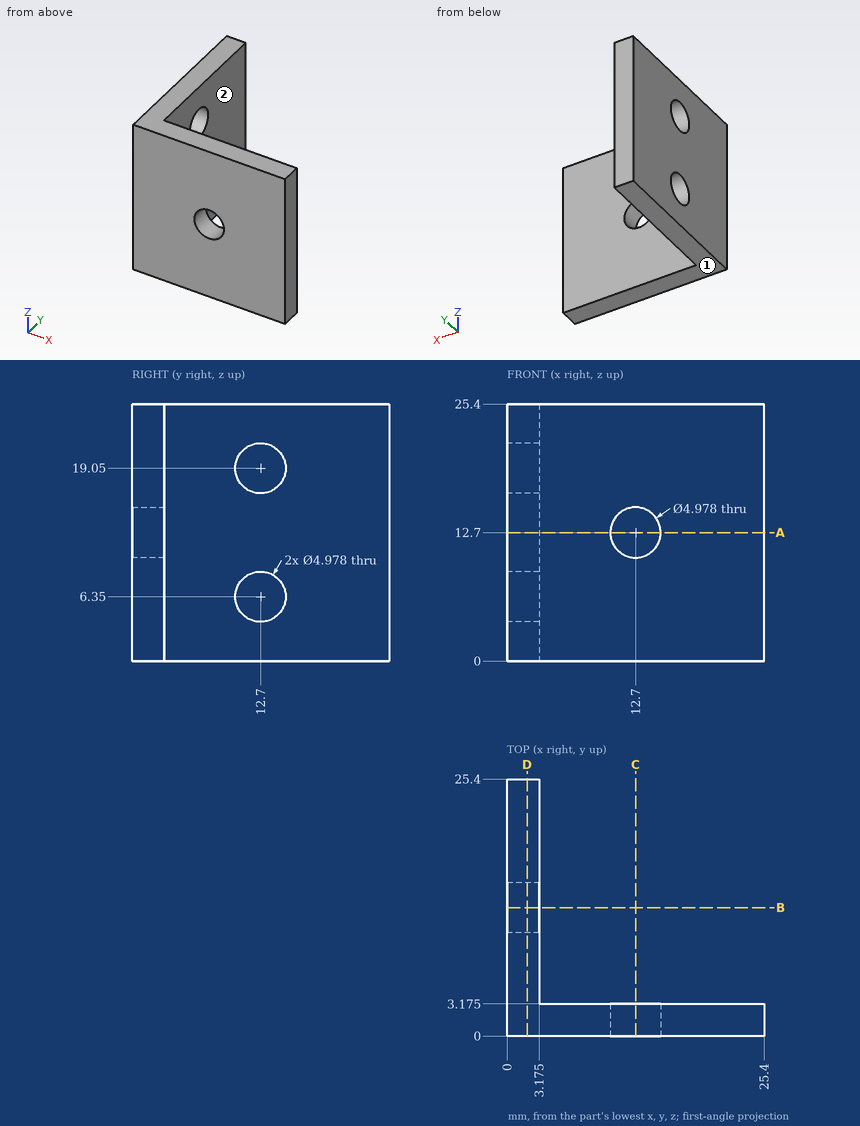
Study the drawing (mm; zero at the part's minimum x, y, z) and answer. A direction names the side the tool comes from. Coordinates: 2 decimals unless noted, no trailing zeros. Loops run counter-clockwise (first coordinate to the right, second up) from the corner with the lowest first, then second, coordinate; pieces in that order, holes last. Notation, with made-up numbers: (-35.5, -5) -> (-6.5, -5) arc R24 cw to (-6.5, 6) -> close; hole circle Ø4 at (15, 49). An arc over 180 degrees is marked (long way). Answer as CSV lines item,"result".
1) Straight lines are drawn through the part: probe 1 along Z at (x, y) = (2.55, 12.7); probe 2 along X at (y, z) = (0.9, 12.7). For each, find the intervals that lie inside material, in ascending order.
A:
probe 1,"z = 0 to 3.86, 8.84 to 16.56, 21.54 to 25.4"
probe 2,"x = 0 to 10.21, 15.19 to 25.4"
2) The part is cut by section D-D (x = 2). Give the vertices of the cut face in (y, z).
A:
outline,"(0, 0) -> (25.4, 0) -> (25.4, 25.4) -> (0, 25.4) -> close; hole circle Ø4.98 at (12.7, 6.35); hole circle Ø4.98 at (12.7, 19.05)"
3) The part is cut by section B-B (y = 12.7). Give the vertices of the cut face in (x, z) (1 decimal).
A:
outline,"(0, 0) -> (3.2, 0) -> (3.2, 3.9) -> (0, 3.9) -> close; (0, 8.8) -> (3.2, 8.8) -> (3.2, 16.6) -> (0, 16.6) -> close; (0, 21.5) -> (3.2, 21.5) -> (3.2, 25.4) -> (0, 25.4) -> close"
4) Flat-ended cylindrical pins translate along their axes: pin 1 (10 mm diameter, centred on y = 21.5, z = 16.5, fed in from +X) (3 decimals); pin 2 (6 mm diameter, centred on x = 6.5, z = 20, fed in from +Y) (3 decimals). Find the tip coordinate at first contact, or state that the pin passes through.
A:
pin 1,"stops at x = 3.175"
pin 2,"stops at y = 3.175"
5) The part is cut by section C-C (x = 12.7). Give the vertices of the cut face in (y, z) (1 decimal).
A:
outline,"(0, 0) -> (3.2, 0) -> (3.2, 10.2) -> (0, 10.2) -> close; (0, 15.2) -> (3.2, 15.2) -> (3.2, 25.4) -> (0, 25.4) -> close"
6) For the marked faces 1 and 2, determine the directions among +Z, -Z, +X, -X, +Y, -Y from which every point of the face is accessible in a straight line to the end or side of a thin tool.
A:
face 1,"-Z, +X, -X, +Y, -Y"
face 2,"+Z, -Z, +X, +Y"
7) The part is cut by section A-A (z = 12.7). Give the vertices of the cut face in (x, y) (1 decimal).
A:
outline,"(0, 0) -> (10.2, 0) -> (10.2, 3.2) -> (3.2, 3.2) -> (3.2, 25.4) -> (0, 25.4) -> close; (15.2, 0) -> (25.4, 0) -> (25.4, 3.2) -> (15.2, 3.2) -> close"
